Verification items for the finished model (mm, model axes). A direction names the side the tool comes from. Give positions to 0.01 mm unless a question says otherwise; leave off trailing zeros. Loops run counter-clockwise (first coordinate to the right, second up) from the corner with the lowest first, then second, coordinate; pieces in that order, holes last. Notation, with made-up numbers: (6.5, 35.5) - (49.5, 35.5) arc R15 cw to (49.5, 61.5) - close; hole circle Ø5 at (4, -18). An arc over 180 degrees is marked (long way). One line per item, written item: value. Start each with the question number.
1. Sectioned sample at D-D (y = 58). Record the cut outline in (x, z).
2. Sectioned sample at C-C (x = 40.5). Record the cut outline in (y, z), plus the area to 3 significant figures.
3. Access from +Z, -Z, +X, -X, +Y, -Y to the whole of each face (thin tool, end or side, straight path). Record for faces 1 (the flat face through (43.9, 33, 7.4)), 2 (the flat face through (68.384, 25.958, 7.395)), 3 (the flat face through (32, 22, 0)), 4 (the flat face through (-20, -3.956, 2)), 5 (the flat face through (78, 57, 4.5)).
4. Sectioned sample at B-B (x = -13). Record the cut outline in (y, z), plus the area to 3 significant figures.
5. Mould release check, pull along Y, two halves, no side actions. Record for faces 6 (the flat face through (53.623, 22.096, 7.395)), 7 (the flat face through (-16, 0, 7)), 8 (the cylindrical face through (81.081, 60.335, 2.218)): pulls with the +Y half, pulls with the -Y half, needs draft (parallel to the pull), parting line crosses it, or undercut.
6. Gauge pin test, flat ends, axial feed: pin 1 (8 mm diameter, centred on x = 54.5, z = 7, fed in from +Y); pin 2 (6 mm diameter, centred on y = 8.5, z = 2.5, fed in from +X); pin 3 (6 mm diameter, centred on y = 41, z = 9, fed in from +X). Record the tip position at first contact, or that the pin passes through.
7. Sectioned sample at A-A (y = 17.5). Record the cut outline in (x, z).
8. Scan lines: L1, parallel to Z at x = 78.5, y = 57; L2, parallel to Y at x = -7.5, z = 2; L3, parallel to X at y = 23, z = 8.75. Record each from-to range of solid material in increasing order. Write a range as [from, to].
from build123d import *

# Parameters (mm, degrees)
BOSS_EXTRUDE1_DEPTH = 15
FILLET1_R           = 5
SKETCH4_W           = 6
SKETCH4_H           = 10
FILLET3_START       = 4.5
FILLET3_DEPTH       = 6
CUT_EXTRUDE1_REACH  = 110.311
CUT_EXTRUDE2_DEPTH  = 20
FILLET4_R           = 0.2


with BuildPart() as part:
    # Sketch1 → Boss-Extrude1 (new body)
    with BuildSketch(Plane.XY):
        with BuildLine():
            Line((0, 0), (60.104076401, 60.104076401))
            ThreePointArc((60.104076401, 60.104076401), (81.317279836, 60.104076401), (81.317279836, 38.890872965))
            Line((81.317279836, 38.890872965), (55.084101547, 12.657694676))
            Line((55.084101547, 12.657694676), (44.518645004, -10))
            Line((44.518645004, -10), (-30, -10))
            Line((-30, -10), (-30, 0))
            Line((-30, 0), (0, 0))
        make_face()
    extrude(amount=BOSS_EXTRUDE1_DEPTH)

    # Fillet1
    fillet1_edges = [part.edges().sort_by_distance(p)[0] for p in [
        (0, 0, 7.5),
    ]]
    fillet(fillet1_edges, radius=FILLET1_R)

    # Cut-Sweep1: sweep along a path in Sketch3
    with BuildLine(Plane.XY.offset(7.5)) as cut_sweep1_path:
        ThreePointArc((81.317279836, 38.890872965), (81.317279836, 60.104076401), (60.104076401, 60.104076401))
    # Sketch4 → Cut-Sweep1 (sweep, cut)
    with BuildSketch(Plane(origin=(60.104076401, 60.104076401, 0), x_dir=(0, 0, -1), z_dir=(-0.7071067811865462, -0.7071067811865489, 0))):
        with Locations((-7.5, 0)):
            Rectangle(SKETCH4_W, SKETCH4_H)
    sweep(path=cut_sweep1_path.line, mode=Mode.SUBTRACT)

    # Fillet3: read off the stored shape, not the designer's step
    # Fillet3 outline → Fillet3 (cut)
    with BuildSketch(Plane.XY.offset(FILLET3_START)):
        with BuildLine():
            add(Edge.make_bspline(
                [(75.193555479, 32.767148608), (79.276038384, 36.849631513), (77.781745931, 42.426406871)],
                knots=[0, 0, 0, 1, 1, 1], degree=2, weights=[1, 0.111111111, 1]))
            Line((75.193555479, 32.767148608), (81.317279836, 38.890872965))
            Line((81.317279836, 38.890872965), (77.781745931, 42.426406871))
        make_face()
        with BuildLine():
            Line((60.104076401, 60.104076401), (53.980352044, 53.980352044))
            add(Edge.make_bspline(
                [(53.980352044, 53.980352044), (58.062834949, 58.062834949), (63.639610307, 56.568542495)],
                knots=[0, 0, 0, 1, 1, 1], degree=2, weights=[1, 0.111111111, 1]))
            Line((63.639610307, 56.568542495), (60.104076401, 60.104076401))
        make_face()
    extrude(amount=FILLET3_DEPTH, mode=Mode.SUBTRACT)

    # Sketch5 → Cut-Extrude1 (cut, up to next)
    with BuildSketch(Plane(origin=(0, 0, 0), x_dir=(-1, 0, 0), z_dir=(0, 0, -1)), mode=Mode.PRIVATE) as cut_extrude1_sk1:
        with BuildLine():
            Line((-65.553913935, 54.654238867), (-21.67846541, 10.778790341))
            ThreePointArc((-21.67846541, 10.778790341), (-21.67846541, 0.465261974), (-31.991993777, 0.465261974))
            Line((-31.991993777, 0.465261974), (-75.867442302, 44.3407105))
            ThreePointArc((-75.867442302, 44.3407105), (-75.867442302, 54.654238867), (-65.553913935, 54.654238867))
        make_face()
    cut_extrude1_tool1 = extrude(cut_extrude1_sk1.sketch, amount=-CUT_EXTRUDE1_REACH, mode=Mode.PRIVATE) & part.part
    add(cut_extrude1_tool1.solids().sort_by_distance((48.772954, 27.55975, 0))[0], mode=Mode.SUBTRACT)

    # Sketch7 → Cut-Extrude2 (cut)
    with BuildSketch(Plane.ZY.offset(30)):
        Polygon((15, -3.955549677), (11.3, -3.955549677), (13.5, -10), (15, -10), align=None)
        Polygon((0, -10), (0, -3.955549677), (3.7, -3.955549677), (1.5, -10), align=None)
    extrude(amount=-CUT_EXTRUDE2_DEPTH, mode=Mode.SUBTRACT)

    # Fillet4
    fillet4_edges = [part.edges().sort_by_distance(p)[0] for p in [
        (-10, -3.955549677, 13.15),
        (-20, -3.955549677, 11.3),
        (-10, -3.955549677, 1.85),
        (-20, -3.955549677, 3.7),
    ]]
    fillet(fillet4_edges, radius=FILLET4_R)


solid = part.part
Results are:
1. outline: (58, 0) - (83.07, 0) - (83.07, 4.5) - (75.97, 4.5) - (75.97, 10.5) - (83.07, 10.5) - (83.07, 15) - (58, 15) - (58, 10.5) - (65.45, 10.5) - (65.45, 4.5) - (58, 4.5) - close
2. outline: (-10, 0) - (8.97, 0) - (8.97, 15) - (-10, 15) - close; (29.6, 0) - (40.5, 0) - (40.5, 15) - (29.6, 15) - close
2. area: 448 mm^2
3. face 1: +Z, -Z
3. face 2: +Z, -Z, +X, -Y
3. face 3: -Z, +X, -X, +Y, -Y
3. face 4: -Z, -X
3. face 5: none
4. outline: (-10, 1.5) - (-4.22, 3.6) arc R0.2 cw to (-3.96, 3.41) - (-3.96, 0) - (0, 0) - (0, 15) - (-3.96, 15) - (-3.96, 11.59) arc R0.2 cw to (-4.22, 11.4) - (-10, 13.5) - close
4. area: 119 mm^2
5. face 6: undercut
5. face 7: pulls with the +Y half
5. face 8: parting line crosses it
6. pin 1: stops at y = 57.62
6. pin 2: stops at x = 54.54
6. pin 3: stops at x = 84.5
7. outline: (17.5, 0) - (28.4, 0) - (28.4, 15) - (17.5, 15) - close; (49.03, 0) - (59.93, 0) - (59.93, 15) - (49.03, 15) - close
8. L1: z = [0, 4.5], [10.5, 15]
8. L2: y = [-10, 0]
8. L3: x = [23, 33.9], [54.53, 65.43]
